CAD build for the part. Positions are in the model's coordinates, mm. A direction names the side the tool comes from. Give positions to 0.01 mm unless a question says otherwise; leave off trailing zeros. Order: outer loops, then holes, each group sorted by start corner. A loop starts at its lowest first (then second) coordinate and runs counter-clockwise, first axis right, second up. Notation, with made-up numbers: (32.5, 38) -> (45.5, 38) arc R9 ccw to (45.5, 50) -> close; hole circle Ø1 at (10.5, -20.5). An arc over 180 degrees is marked (long way). Use one line per item in the form item = value. Start each with the question number.
1) Mould opens along X. For faces 6 (the face through (-0.13, 63.42, -0.03)), 7 (the face through (4.77, 47.86, 0.5)), 8 (the face through (2.2, 38.001, 2.1)) say: pulls with the +X half, pulls with the -X half, needs draft (parallel to the pull), parting line crosses it, or undercut.
2) Cut at B-B, the plane y = 57.5. Give the cut face in (x, z), and give its area (3 significant figures).
3) Probe line 1 (X direction, y = 39, z = 3.75); line 2 (X direction, y = 45.5, z = 4.5); line 3 (Y direction, x = -6, z = -0.5). List the from-to ranges inside material, lowest first.
4) Cut at C-C, the plane y = 43. Give the cut face in (x, z).
5) Tool access for faces 1 (the face through (-0.1, 63.61, 0.63)), 2 (the face through (-4.186, 71.654, 3.559)), 3 (the face through (-3.067, 59, 2)), 4 (the face through (1.43, 46.45, 5.14)), 5 (the face through (-1.474, 46.875, 3.352)): list every direction of +Z, -Z, +X, -X, +Y, -Y with a clear straight run to the whole face (end or side of a thin tool).
6) Cut at A-A, the plane x = 0. State how many separate pieces and enclosed holes the cut face has, and give its area (3 significant figures).
7) Drop flat-ended pins along their axis: P1, Ø2, axis at y = 56, z = -0.5, coming from the -X side; P2, Ø3.5, axis at x = 0, z = 2, coming from the +Y side; P3, Ø2.5, axis at x = 0, y = 46, coming from the +Z side; P4, Ø2, axis at x = 7.5, z = -1.5, coming from the +Y side. Give the stop position or say it passes through.
from build123d import *

# Parameters (mm, degrees)
SKETCH1_W                    = 30
SKETCH1_H                    = 30
BOSS_EXTRUDE1_DEPTH          = 3
SKETCH2_R                    = 5
BOSS_EXTRUDE2_DEPTH          = 55
CUT_EXTRUDE2_DEPTH           = 55
CUT_EXTRUDE3_DEPTH           = 7
CUT_EXTRUDE3_TAPER           = -9
CUT_EXTRUDE3_OTHER_WAY_DEPTH = 2
CUT_EXTRUDE4_DEPTH           = 7
CUT_EXTRUDE4_TAPER           = -9
CUT_EXTRUDE4_OTHER_WAY_DEPTH = 2
CUT_EXTRUDE4_OTHER_WAY_TAPER = -9
SKETCH11_W                   = 42.456870871
SKETCH11_H                   = 39.887112897
CUT_EXTRUDE5_DEPTH           = 16
CUT_EXTRUDE5_DEPTH_BACK      = 16
SKETCH12_W                   = 30
SKETCH12_H                   = 30
BOSS_EXTRUDE3_DEPTH          = 3
SKETCH13_W                   = 6.134758984
SKETCH13_H                   = 3.5
REVOLVE3_ANGLE               = 90
SKETCH14_W                   = 34.327932252
SKETCH14_H                   = 34.043423274
CUT_EXTRUDE6_DEPTH           = 3.3
SKETCH17_R                   = 2
CUT_EXTRUDE7_DEPTH           = 18
SKETCH18_R                   = 1.5
CUT_EXTRUDE8_DEPTH           = 8
CUT_EXTRUDE8_DEPTH_BACK      = 4


with BuildPart() as part:
    # Sketch1 → Boss-Extrude1 (new body)
    with BuildSketch(Plane(origin=(0, 0, 0), x_dir=(1, 0, 0), z_dir=(0, 1, 0))):
        Rectangle(SKETCH1_W, SKETCH1_H)
    extrude(amount=BOSS_EXTRUDE1_DEPTH)

    # Sketch2 → Boss-Extrude2 (add)
    with BuildSketch(Plane(origin=(0, 3, 0), x_dir=(1, 0, 0), z_dir=(0, 1, 0))):
        with Locations((0, -2)):
            Circle(SKETCH2_R)
    extrude(amount=BOSS_EXTRUDE2_DEPTH)

    # Sketch4 → Revolve1 (revolve)
    with BuildSketch(Plane(origin=(0, 0, 0), x_dir=(0, 0, -1), z_dir=(1, 0, 0))):
        Polygon((2.995694392, 58.01182956), (0.17661653, 56.98576913), (-1.106821781, 63.435791308), (-0.16712916, 63.777811451), align=None)
    revolve(axis=Axis((0, 68.333514617, -2.116247015), (0, -0.342020143, 0.939692621)))

    # Sketch5 → Cut-Extrude2 (cut)
    with BuildSketch(Plane(origin=(0, 7.748892564, -21.289907346), x_dir=(1, 0, 0), z_dir=(0, 0.342020143, -0.939692621))):
        Polygon((-3, -65.291475968), (-6.572175958, -75.105948751), (6.572175958, -75.105948751), (3, -65.291475968), align=None)
    extrude(amount=-CUT_EXTRUDE2_DEPTH, mode=Mode.SUBTRACT)

    # Sketch6 → Cut-Extrude3 (cut)
    with BuildSketch(Plane(origin=(37.638193634, 42.150337699, 15.341468287), x_dir=(0, -0.342020143, 0.939692621), z_dir=(0.64278761, 0.71984631, 0.26200263))):
        Polygon((-22.656246175, -42.076297889), (-21.656246175, -42.076297889), (-22.656246175, -39.576297889), align=None)
        Polygon((-19.616275943, -42.076297889), (-19.616275943, -39.576297889), (-20.616275943, -42.076297889), align=None)
    extrude(amount=-CUT_EXTRUDE3_DEPTH, taper=CUT_EXTRUDE3_TAPER, mode=Mode.SUBTRACT)

    # Sketch6 → Cut-Extrude3 other way (cut)
    with BuildSketch(Plane(origin=(37.638193634, 42.150337699, 15.341468287), x_dir=(0, -0.342020143, 0.939692621), z_dir=(0.64278761, 0.71984631, 0.26200263))):
        Polygon((-22.656246175, -42.076297889), (-21.656246175, -42.076297889), (-22.656246175, -39.576297889), align=None)
        Polygon((-19.616275943, -42.076297889), (-19.616275943, -39.576297889), (-20.616275943, -42.076297889), align=None)
    extrude(amount=CUT_EXTRUDE3_OTHER_WAY_DEPTH, mode=Mode.SUBTRACT)

    # Sketch8 → Cut-Extrude4 (cut)
    with BuildSketch(Plane(origin=(-37.638193634, 42.150337699, 15.341468287), x_dir=(0, 0.342020143, -0.939692621), z_dir=(0.64278761, -0.71984631, -0.26200263))):
        Polygon((22.656246175, 42.076297889), (21.656246175, 42.076297889), (22.656246175, 39.576297889), align=None)
        Polygon((20.656246175, 42.076297889), (19.656246175, 42.076297889), (19.656246175, 39.576297889), align=None)
    extrude(amount=CUT_EXTRUDE4_DEPTH, taper=CUT_EXTRUDE4_TAPER, mode=Mode.SUBTRACT)

    # Sketch8 → Cut-Extrude4 other way (cut)
    with BuildSketch(Plane(origin=(-37.638193634, 42.150337699, 15.341468287), x_dir=(0, 0.342020143, -0.939692621), z_dir=(0.64278761, -0.71984631, -0.26200263))):
        Polygon((22.656246175, 42.076297889), (21.656246175, 42.076297889), (22.656246175, 39.576297889), align=None)
        Polygon((20.656246175, 42.076297889), (19.656246175, 42.076297889), (19.656246175, 39.576297889), align=None)
    extrude(amount=-CUT_EXTRUDE4_OTHER_WAY_DEPTH, taper=CUT_EXTRUDE4_OTHER_WAY_TAPER, mode=Mode.SUBTRACT)

    # Sketch11 → Cut-Extrude5 (cut, two sides)
    with BuildSketch(Plane(origin=(0, 0, 0), x_dir=(0, 0, -1), z_dir=(1, 0, 0))) as cut_extrude5_sk:
        with Locations((2.849079493, 17.75767337)):
            Rectangle(SKETCH11_W, SKETCH11_H)
    extrude(amount=CUT_EXTRUDE5_DEPTH, mode=Mode.SUBTRACT)
    extrude(cut_extrude5_sk.sketch, amount=-CUT_EXTRUDE5_DEPTH_BACK, mode=Mode.SUBTRACT)

    # Sketch12 → Boss-Extrude3 (add)
    with BuildSketch(Plane.XZ.offset(-37.701229818)):
        Rectangle(SKETCH12_W, SKETCH12_H)
    extrude(amount=BOSS_EXTRUDE3_DEPTH)

    # Sketch13 → Revolve3 (revolve)
    with BuildSketch(Plane(origin=(0, 58, 0), x_dir=(1, 0, 0), z_dir=(0, 1, 0))):
        with Locations((0, -1.75)):
            Rectangle(SKETCH13_W, SKETCH13_H)
    revolve(axis=Axis((-3.067379492, 58, 0), (-1, 0, 0)), revolution_arc=REVOLVE3_ANGLE)

    # Sketch14 → Cut-Extrude6 (cut)
    with BuildSketch(Plane.XZ.offset(-34.701229818)):
        with Locations((-1.184585751, 0.782917941)):
            Rectangle(SKETCH14_W, SKETCH14_H)
    extrude(amount=-CUT_EXTRUDE6_DEPTH, mode=Mode.SUBTRACT)

    # Sketch17 → Cut-Extrude7 (cut)
    with BuildSketch(Plane.XZ.offset(-38.001229818)):
        with Locations((0, 2)):
            Circle(SKETCH17_R)
    extrude(amount=-CUT_EXTRUDE7_DEPTH, mode=Mode.SUBTRACT)

    # Sketch18 → Cut-Extrude8 (cut, two sides)
    with BuildSketch(Plane.XY) as cut_extrude8_sk:
        with Locations((0, 46.001229818)):
            Circle(SKETCH18_R)
    extrude(amount=CUT_EXTRUDE8_DEPTH, mode=Mode.SUBTRACT)
    extrude(cut_extrude8_sk.sketch, amount=-CUT_EXTRUDE8_DEPTH_BACK, mode=Mode.SUBTRACT)


solid = part.part
Result:
q1.face_6 = undercut
q1.face_7 = parting line crosses it
q1.face_8 = needs draft
q2.outline = circle Ø10 at (0, 2)
q2.area = 78.5 mm²
q3.line_1 = -4.68 to -0.97, 0.97 to 4.68
q3.line_2 = -4.33 to -1.41, 1.41 to 4.33
q3.line_3 = 59.23 to 63.59
q4.outline = circle Ø10 at (0, 2); hole circle Ø4 at (0, 2)
q5.face_1 = none
q5.face_2 = +Z, +Y
q5.face_3 = +Z
q5.face_4 = +Z, -Z
q5.face_5 = -Y
q6.separate_pieces = 3
q6.enclosed_holes = 0
q6.area = 130 mm²
q7.P1 = -4.77
q7.P2 = 63.8
q7.P3 = through
q7.P4 = 64.11
